Drawing for the job (mm, zero at the part's lowest x, y, z). A direction names the side the tool comes from. Round coordinates to 2 decimals unless told otherwise and drop trailing zeros. Loops run counter-clockwise (first coordinate to the right, second up) from the corner with the lowest first, then second, coordinate; pieces in that order, holes last.
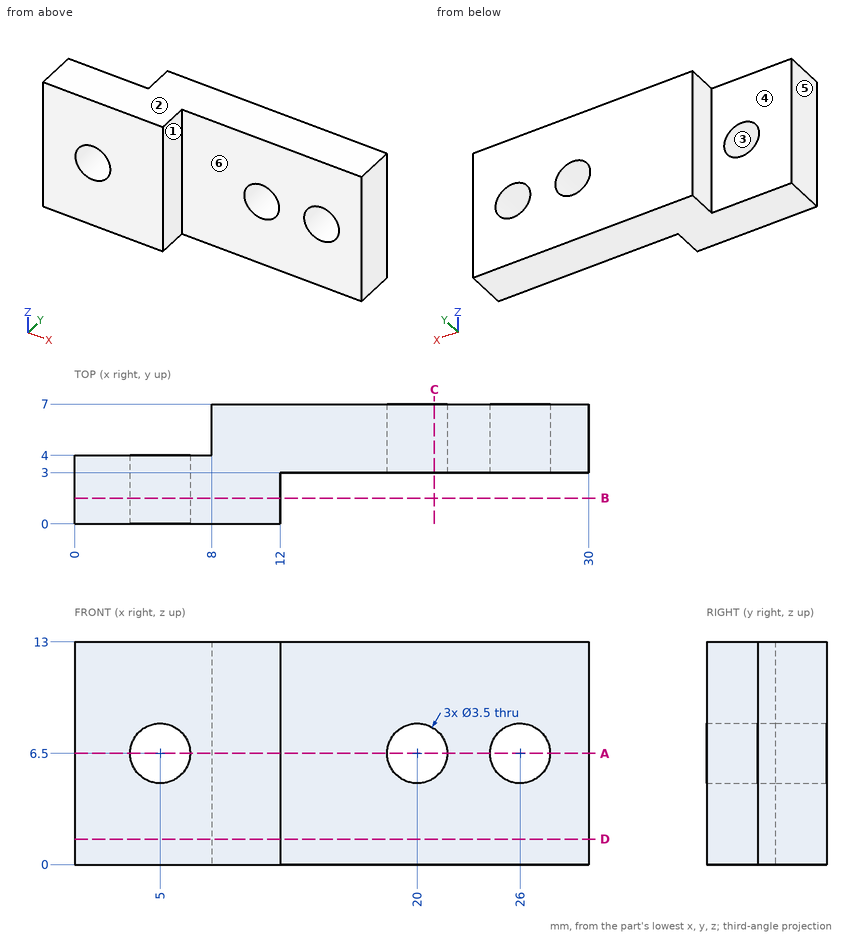
Q1. Slice it at D-D on z = 1.5. Give the cut face in (x, y).
Q2. Flat gauge pins, fed straight in: P1, Ø1.5, axis at y = 2, z = 10, coming from the +X side; P2, Ø1.5, axis at y = 5, z = 7, coming from the -X side; P3, Ø4.5, axis at x = 26, z = 6.5, coming from the -Y side. Where does each tip first touch, or does it go through?
Q3. Pull direction Z, two halves, no side cores. Call the marked faces 1, 2 and 3: pulls with the +Z half, pulls with the -Z half, needs draft (parallel to the pull), parting line crosses it, or undercut.
Q4. Slice it at A-A on z = 6.5. Give the cut face in (x, y), plus the area to 3 significant figures.
Q5. Probe line 1 (X direction, y = 6, z = 6.5); line 2 (X direction, y = 1.1, z = 6.5); line 3 (Z direction, x = 20, y = 5.3). List the from-to ranges inside material, lowest first.
Q6. Slice it at B-B on y = 1.5. Give the cut face in (x, z).
Q7. Slice it at C-C on x = 21. Give the cut face in (y, z), plus the area to 3 significant figures.
Q8. Tool access for the marked faces 4, 5 and 6: list every direction of +Z, -Z, +X, -X, +Y, -Y with a clear straight run to the whole face (end or side of a thin tool).
Reply:
1. outline: (0, 0) - (12, 0) - (12, 3) - (30, 3) - (30, 7) - (8, 7) - (8, 4) - (0, 4) - close
2. P1: stops at x = 12
2. P2: stops at x = 8
2. P3: stops at y = 3
3. face 1: needs draft
3. face 2: pulls with the +Z half
3. face 3: undercut
4. outline: (0, 0) - (3.25, 0) - (3.25, 4) - (0, 4) - close; (6.75, 0) - (12, 0) - (12, 3) - (18.25, 3) - (18.25, 7) - (8, 7) - (8, 4) - (6.75, 4) - close; (21.75, 3) - (24.25, 3) - (24.25, 7) - (21.75, 7) - close; (27.75, 3) - (30, 3) - (30, 7) - (27.75, 7) - close
4. area: 90.0 mm2
5. line 1: x = 8 to 18.25, 21.75 to 24.25, 27.75 to 30
5. line 2: x = 0 to 3.25, 6.75 to 12
5. line 3: z = 0 to 4.75, 8.25 to 13
6. outline: (0, 0) - (12, 0) - (12, 13) - (0, 13) - close; hole circle Ø3.5 at (5, 6.5)
7. outline: (3, 0) - (7, 0) - (7, 5.06) - (3, 5.06) - close; (3, 7.94) - (7, 7.94) - (7, 13) - (3, 13) - close
7. area: 40.5 mm2
8. face 4: +Z, -Z, -X, +Y
8. face 5: +Z, -Z, -X, +Y, -Y
8. face 6: +Z, -Z, +X, -Y
